Source: CAD feature listing. Evaluate the final solid. Frame: model axes, mm. Face numbers are marked on the shaded views. A direction names the side the tool comes from. Coordinates: 2 decimals unless noted, no trailing zeros. Write each loop counter-clockwise with the first axis right and the second up, starting at its lowest first coordinate (ties: lowest second). Pieces come first, ordered by that corner, then holes. Notation, with made-up numbers: (89, 52.25) -> (123, 52.25) arc R23 cw to (123, 85.25) -> close; hole circle Ø2 at (1.5, -22.75). An arc over 180 degrees is marked (long way). One line per item, written item: value. Start each with the question number.
1. Section query B-B, the plane x = 40.5. Output: boundary loops of the cut face in (y, z), and give its area (3 significant figures).
2. First-contact query: P1, Ø8, axis at x = 30.5, y = 27.5, coming from the -Z side; P2, Ø3.5, axis at x = 9.5, z = -9.5, coming from the -Y side (3 decimals); P3, Ø15, axis at x = 17, z = -17, coming from the +Y side; P4, Ø6, axis at y = 35.5, z = -27, coming from the +X side. Flat tips, straight axial feed; report the tip coordinate or a pass-through.
3. Line query: line 1 (X direction, y = 2.6, z = -40.5); line 2 (Y direction, x = 5.5, z = -42.5); line 3 (Z direction, x = 20, y = 36). Output: solid intervals per line, ascending.
4. Section query C-C, the plane y = 34.5. Output: boundary loops of the cut face in (x, z), and give its area (3 significant figures).
5. Access query for the marked faces 1, 2 and 3. Directions: +Z, -Z, +X, -X, +Y, -Y. A direction counts if a zero-diameter tool reaches every point of the face in a straight line with its end or side. Return the directions, or none.
6. Section query D-D, the plane x = 15. Output: boundary loops of the cut face in (y, z).
7. Section query A-A, the plane z = -40.5. Output: boundary loops of the cut face in (x, y), and give its area (3 significant figures).
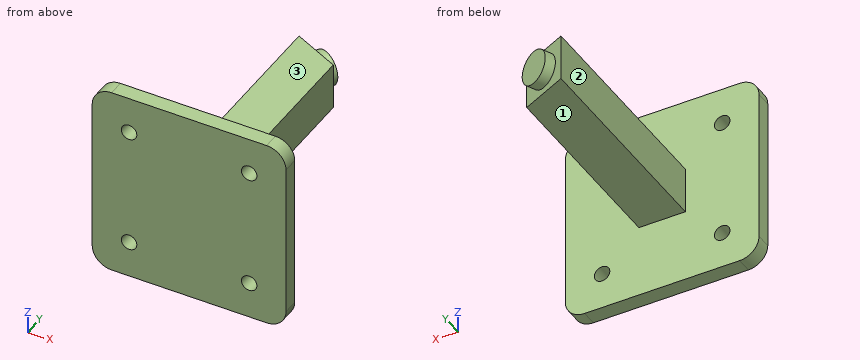
from build123d import *

# Parameters (mm, degrees)
SKETCH1_R           = 2
BOSS_EXTRUDE1_DEPTH = 4
SKETCH3_W           = 12
SKETCH3_H           = 12
BOSS_EXTRUDE3_DEPTH = 51.3
BOSS_EXTRUDE4_DEPTH = 12
SKETCH6_R           = 4.45
BOSS_EXTRUDE5_DEPTH = 2.8


with BuildPart() as part:
    # Sketch1 → Boss-Extrude1 (new body)
    with BuildSketch(Plane(origin=(0, 0, 0), x_dir=(1, 0, 0), z_dir=(0, 1, 0))):
        with BuildLine():
            Line((5, 0), (45, 0))
            ThreePointArc((45, 0), (48.535533906, 1.464466094), (50, 5))
            Line((50, 5), (50, 45))
            ThreePointArc((50, 45), (48.535533906, 48.535533906), (45, 50))
            Line((45, 50), (5, 50))
            ThreePointArc((5, 50), (1.464466094, 48.535533906), (0, 45))
            Line((0, 45), (0, 5))
            ThreePointArc((0, 5), (1.464466094, 1.464466094), (5, 0))
        make_face()
        with Locations(Location((9.5, 9.5, 0), (0, 0, 270))):
            Circle(SKETCH1_R, mode=Mode.SUBTRACT)
        with Locations(Location((9.5, 40.5, 0), (0, 0, 270))):
            Circle(SKETCH1_R, mode=Mode.SUBTRACT)
        with Locations(Location((40.5, 40.5, 0), (0, 0, 270))):
            Circle(SKETCH1_R, mode=Mode.SUBTRACT)
        with Locations(Location((40.5, 9.5, 0), (0, 0, 270))):
            Circle(SKETCH1_R, mode=Mode.SUBTRACT)
    extrude(amount=BOSS_EXTRUDE1_DEPTH)

    # Sketch3 → Boss-Extrude3 (add)
    with BuildSketch(Plane(origin=(0, 4, 0), x_dir=(1, 0, 0), z_dir=(0, 1, 0))):
        with Locations((25, 25)):
            Rectangle(SKETCH3_W, SKETCH3_H)
    extrude(amount=BOSS_EXTRUDE3_DEPTH)

    # Sketch5 → Boss-Extrude4 (add)
    with BuildSketch(Plane.XY.offset(-19)):
        Polygon((31, 55.3), (19, 60.895691898), (19, 55.3), align=None)
    extrude(amount=-BOSS_EXTRUDE4_DEPTH)

    # Sketch6 → Boss-Extrude5 (add)
    with BuildSketch(Plane(origin=(26.717920902, 57.296766276, 0), x_dir=(0.9063077870366527, -0.4226182617406934, 0), z_dir=(0.42261826174069345, 0.9063077870366528, 0))):
        with Locations(Location((-1.89551599, 25, 0), (0, 0, 180))):
            Circle(SKETCH6_R)
    extrude(amount=BOSS_EXTRUDE5_DEPTH)


solid = part.part
Computed values:
1. outline: (0, -50) -> (4, -50) -> (4, -42.5) -> (0, -42.5) -> close; (0, -38.5) -> (4, -38.5) -> (4, -11.5) -> (0, -11.5) -> close; (0, -7.5) -> (4, -7.5) -> (4, 0) -> (0, 0) -> close
1. area: 168 mm²
2. P1: stops at z = -31
2. P2: passes through
2. P3: stops at y = 60.9
2. P4: stops at x = 31
3. line 1: x = 0 to 7.5, 11.5 to 38.5, 42.5 to 50
3. line 2: y = 0 to 4
3. line 3: z = -31 to -19
4. outline: (19, -31) -> (31, -31) -> (31, -19) -> (19, -19) -> close
4. area: 144 mm²
5. face 1: -Z, +X, -X, +Y
5. face 2: +Z, -Z, -X, +Y
5. face 3: +Z, +X, -X, +Y
6. outline: (0, -50) -> (4, -50) -> (4, 0) -> (0, 0) -> close
7. outline: (0, 0) -> (7.5, 0) -> (7.5, 4) -> (0, 4) -> close; (11.5, 0) -> (38.5, 0) -> (38.5, 4) -> (11.5, 4) -> close; (42.5, 0) -> (50, 0) -> (50, 4) -> (42.5, 4) -> close
7. area: 168 mm²
